Geometry: final body of the model. Coordinates: model frame, mm. Give positions to 0.01 mm unless a question says otherwise; leave off trailing zeros. Write each loop counter-clockwise with the first axis right and the second up, starting at its lowest first coordinate (ties: lowest second). Pieces come first, ordered by that corner, then holes. Notation, with made-up numbers: M 21.5,10.25 L 74.5,10.25 A11 cw 74.5,26.25 Z; hole C 6,35.5 d2. An arc over 180 degrees is marked long. Use one line per item in the form item = value. Start each with the question number.
Item 1: Pull-direction query (Y, two-part tool) for faces 1 (the cylindrical face through (-1.5, 0.07, 4.56)), 2 (the flat face through (-1, 1, 11.25)), 3 (the flat face through (0, 0, 10.25)); classes: released by +Y, released by -Y, zero draft, split by the parting line, or undercut.
Item 2: Section query C-C on z = 6.25. Return loops of the section in (x, y).
Item 3: Contact query for flat-ended pins moving along their axis: P1, Ø0.6, axis at y = -1, z = 11, coming from the -X side; P2, Ø1.5, axis at y = 1, z = 5, coming from the -X side; P3, Ø1, axis at x = 1, z = 6.5, coming from the +Y side. Output: stop coordinate, or through.
Item 4: Material intervals for line 1 along X through (y, z) = (0.05, 3.75); line 2 along Y through (x, z) = (-1.2, 10.75); line 3 along Z through (x, y) = (-0.2, 0.1), sorted ascending. Write a range as from..to.
from build123d import *

# Parameters (mm, degrees)
F0_R     = 1.5
F1_DEPTH = 9.25
F2_R     = 2.7
F3_DEPTH = 2
F5_DEPTH = 1
F6_R     = 0.25
F7_R     = 0.99999


# Not quite as in the source:
# - a fillet or chamfer is up to 0.001 mm smaller than in the source, because OpenCascade refuses the exact size


with BuildPart() as f1:
    # F0 (on Top) → F1 (new body)
    with BuildSketch(Plane.XY):
        Circle(F0_R)
    extrude(amount=F1_DEPTH)

    # F2 (on face) → F3 (join)
    with BuildSketch(Plane.XY.offset(9.25)):
        Circle(F2_R)
    extrude(amount=F3_DEPTH)

    # F4 (on face) → F5 (cut)
    with BuildSketch(Plane.XY.offset(11.25)):
        Polygon((0.5, 1.5), (-0.5, 1.5), (-0.5, 0.5), (-1.5, 0.5), (-1.5, -0.5), (-0.5, -0.5), (-0.5, -1.5), (0.5, -1.5), (0.5, -0.5), (1.5, -0.5), (1.5, 0.5), (0.5, 0.5), align=None)
    extrude(amount=-F5_DEPTH, mode=Mode.SUBTRACT)

    # F6
    f6_edges = [f1.edges().sort_by_distance(p)[0] for p in [
        (0, 1.5, 10.25),
        (-0.5, 1, 10.25),
        (-1, 0.5, 10.25),
        (-1.5, 0, 10.25),
        (-1, -0.5, 10.25),
        (-0.5, -1, 10.25),
        (0, -1.5, 10.25),
        (0.5, -1, 10.25),
        (1, -0.5, 10.25),
        (1.5, 0, 10.25),
        (1, 0.5, 10.25),
        (0.5, 1, 10.25),
    ]]
    fillet(f6_edges, radius=F6_R)

    # F7 (radius 1 in the source; OpenCascade refuses exactly that, so slightly less here)
    f7_edges = [f1.edges().sort_by_distance(p)[0] for p in [
        (2.7, 0, 10.25),
        (-2.7, 0, 9.25),
        (-2.7, 0, 11.25),
    ]]
    fillet(f7_edges, radius=F7_R)


solid = f1.part
Answer sheet:
q1.face_1 = split by the parting line
q1.face_2 = zero draft
q1.face_3 = undercut
q2.outline = C 0,0 d3
q3.P1 = -2.43
q3.P2 = -1.48
q3.P3 = 1.41
q4.line_1 = -1.5..1.5
q4.line_2 = -2.27..-0.5, 0.5..2.27
q4.line_3 = 0..10.25
